Input: part model. Units: mm. Frame: model coordinates. Face numbers are marked on the shaded views. Round coordinates to 2 decimals unless told otherwise and drop trailing zeros. Order: outer loops, then holes, each group sorted by start corner. A loop starts at its lowest first (then second) coordinate and runs counter-clockwise, first axis right, second up. Notation, with made-up numbers: M 24,15 L 80,15 A11 cw 80,28 Z; hole C 60.25,74.5 d4. An arc over 180 degrees is marked long. One line per question, with ' | ' between items.
```python
from build123d import *

# Parameters (mm, degrees)
SKETCH1_W             = 38.1
SKETCH1_H             = 38.1
SKETCH1_W_2           = 34.925
SKETCH1_H_2           = 34.925
EXTRUDE_THIN1_DEPTH   = 152.4
BOSS_EXTRUDE1_DEPTH   = 1.5875
BOSS_EXTRUDE2_START   = 34.925
BOSS_EXTRUDE2_DEPTH   = 1.5875
F_4_CLEARANCE_HOLE1_D = 3.2639


# Read off the part's stored shape, not the designer's step: Boss-Extrude2
with BuildPart() as part:
    # Sketch1 → Extrude-Thin1 (new, symmetric)
    with BuildSketch(Plane(origin=(0, 0, 0), x_dir=(1, 0, 0), z_dir=(0, 1, 0))):
        Rectangle(SKETCH1_W, SKETCH1_H)
        Rectangle(SKETCH1_W_2, SKETCH1_H_2, mode=Mode.SUBTRACT)
    extrude(amount=EXTRUDE_THIN1_DEPTH, both=True)

    # Sketch3 → Boss-Extrude1 (add)
    with BuildSketch(Plane(origin=(-17.4625, 0, 0), x_dir=(0, 0, -1), z_dir=(1, 0, 0))):
        with BuildLine():
            Line((-19.05, 152.4), (19.05, 152.4))
            ThreePointArc((19.05, 152.4), (19.552790503, 154.529854749), (20.955, 156.21))
            ThreePointArc((20.955, 156.21), (22.062069471, 159.754023157), (19.05, 161.925))
            Line((19.05, 161.925), (-19.05, 161.925))
            ThreePointArc((-19.05, 161.925), (-22.062069471, 159.754023157), (-20.955, 156.21))
            ThreePointArc((-20.955, 156.21), (-19.552790503, 154.529854749), (-19.05, 152.4))
        make_face()
    extrude(amount=-BOSS_EXTRUDE1_DEPTH)

    # Boss-Extrude2 outline → Boss-Extrude2 (add)
    with BuildSketch(Plane(origin=(-17.4625, 0, 0), x_dir=(0, 0, -1), z_dir=(1, 0, 0)).offset(BOSS_EXTRUDE2_START)):
        with BuildLine():
            Line((19.05, 161.925), (-19.05, 161.925))
            ThreePointArc((-19.05, 161.925), (-22.062069471, 159.754023157), (-20.955, 156.21))
            ThreePointArc((-20.955, 156.21), (-19.552790503, 154.529854749), (-19.05, 152.4))
            Line((-19.05, 152.4), (19.05, 152.4))
            ThreePointArc((19.05, 152.4), (19.552790503, 154.529854749), (20.955, 156.21))
            ThreePointArc((20.955, 156.21), (22.062069471, 159.754023157), (19.05, 161.925))
        make_face()
    extrude(amount=BOSS_EXTRUDE2_DEPTH)

    # #4 Clearance Hole1 (through all)
    with Locations(Plane.ZY.offset(19.05)):
        with Locations((-19.05, 158.75), (19.05, 158.75)):
            Hole(F_4_CLEARANCE_HOLE1_D / 2)


solid = part.part
```
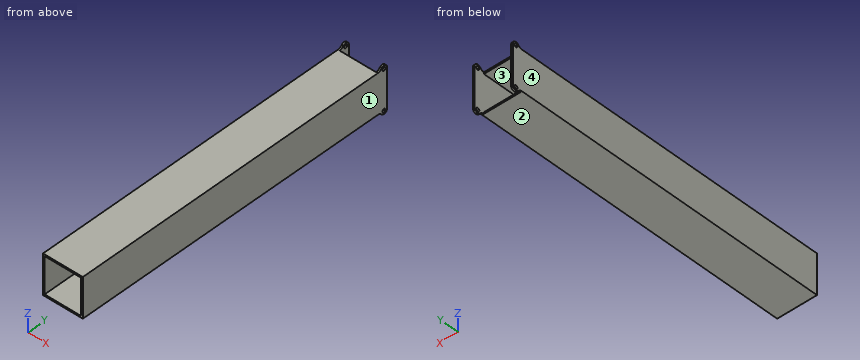
Item 1: Section query B-B, the plane y = -11. Return loops of the section in (x, z), plus the area to 3 significant figures.
Report:
outline: M -19.05,-19.05 L 19.05,-19.05 L 19.05,19.05 L -19.05,19.05 Z; hole M -17.46,-17.46 L 17.46,-17.46 L 17.46,17.46 L -17.46,17.46 Z | area: 232 mm²
Item 2: Mould query, pull axis X, two halves, no side actions, for the marked faces 1, 2, 3 and 4. Classes: +X half, -X half, draft (parallel to the pull), parting line (faces both ways), or undercut.
Report:
face 1: +X half | face 2: draft | face 3: undercut | face 4: -X half
Item 3: Section query C-C, the plane x = -7.5. Return loops of the section in (y, z), plus the area to 3 significant figures.
Report:
outline: M -152.4,-19.05 L 152.4,-19.05 L 152.4,-17.46 L -152.4,-17.46 Z; M -152.4,17.46 L 152.4,17.46 L 152.4,19.05 L -152.4,19.05 Z | area: 968 mm²
Item 4: First-contact query: pin 1 (5 mm diameter, centred on y = 158.75, z = 19.05, fed in from +X); pin 2 (10.5 mm diameter, centred on x = -5.5, y = -28.5, fed in from -Z); pin 3 (2 mm diameter, centred on y = 158.75, z = -19.05, fed in from -X); pin 4 (1.3 mm diameter, centred on x = 1.5, z = 18.5, fed in from +Y). Flat tips, straight axial feed; report the tip coordinate or a pass-through.
Report:
pin 1: x = 19.05 | pin 2: z = -19.05 | pin 3: through | pin 4: y = 152.4
Item 5: Line query: line 1 along Z through (x, y) = (-18.5, 158.75) (3 decimals); line 2 along X through (y, z) = (97, 15.5). Output: solid intervals per line, ascending. Write a range as from..to.
Report:
line 1: -22.225..-20.682, -17.418..17.418, 20.682..22.225 | line 2: -19.05..-17.46, 17.46..19.05
